from build123d import *

# Parameters (mm, degrees)
F1_DEPTH = 12.7
F2_R     = 5.08
F4_D     = 25.4
F4_DEPTH = 6.35
F4_TIP   = 7.6309298617


# Not quite as in the source:
# - a feature names something its author has since deleted; it is built from what else it names


with BuildPart() as f1:
    # F0 (on Right) → F1 (new body)
    with BuildSketch(Plane.YZ):
        with BuildLine():
            ThreePointArc((-15.875, 0), (0, -15.875), (15.875, 0))
            ThreePointArc((15.875, 0), (0, 15.875), (-15.875, 0))
        make_face()
        with BuildLine():
            Line((15.875, -50.8), (15.875, 0))
            ThreePointArc((15.875, 0), (0, -15.875), (-15.875, 0))
            Line((-15.875, 0), (-15.875, -50.8))
            ThreePointArc((-15.875, -50.8), (0, -34.925), (15.875, -50.8))
        make_face()
        with BuildLine():
            ThreePointArc((-15.875, -50.8), (0, -66.675), (15.875, -50.8))
            ThreePointArc((15.875, -50.8), (0, -34.925), (-15.875, -50.8))
        make_face()
    extrude(amount=F1_DEPTH)

    # F2
    f2_edges = [f1.edges().sort_by_distance(p)[0] for p in [
        (12.7, 0, 15.875),
        (12.7, -15.875, -25.4),
        (12.7, 0, -66.675),
        (12.7, 15.875, -25.4),
    ]]
    fillet(f2_edges, radius=F2_R)

    # F4
    with Locations(Plane(origin=(0, 0, 0), x_dir=(0, -1, 0), z_dir=(-1, 0, 0))):
        with Locations((0, 0)):
            Hole(F4_D / 2, depth=F4_DEPTH)
            with Locations((0, 0, -(F4_DEPTH + F4_TIP / 2))):  # 118° drill point
                Cone(0, F4_D / 2, F4_TIP, mode=Mode.SUBTRACT)


solid = f1.part
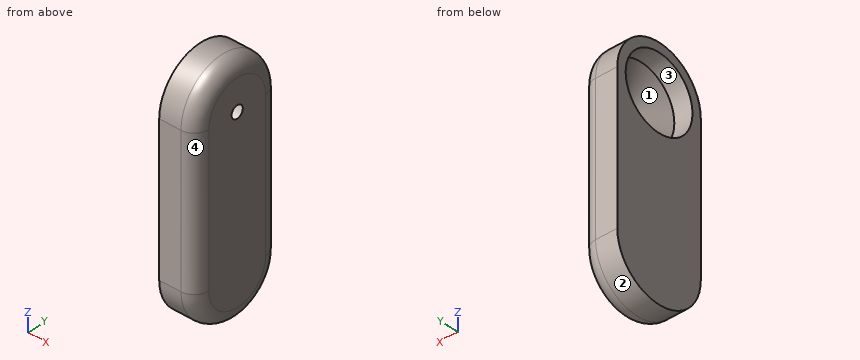
The listing builds one solid part. Answer for the finished solid, in the listing's coordinates (mm). Face numbers are marked on the shaded views. Round coordinates to 2 decimals unless told otherwise and drop trailing zeros. Order: outer loops, then holes, each group sorted by start corner. A loop starts at its lowest first (then second) coordinate and runs counter-clockwise, first axis right, second up. Notation, with made-up numbers: (34.25, 64.5) - (68.25, 64.5) arc R19 cw to (68.25, 100.5) - close; hole circle Ø11 at (88, 46.25). An arc over 180 degrees is marked (long way). Write item = value, one per line. Start each with the question number.
1) Given pin 1 (3 mm diameter, centred on x = 9, y = -3, fed in from -Z); pin 2 (5 mm diameter, centred on x = 8.5, y = 0, fed in from +Z) (3 decimals); pin 3 (4 mm diameter, centred on x = 10.5, z = -33, fed in from +Y), each flat-ended and moving along its own axis, determine where each tip first touches the part or whether it passes through.
2) Section B-B, the plane z = -40 is taken. Write down the section's boundary in (x, y) (3 decimals).
3) Straight lines are drawn through the part: L1, parallel to Y at x = 3, z = 0 (3 decimals); L2, parallel to Z at x = 4.5, y = 0 (3 decimals); L3, parallel to Y at x = 8, z = 2.5. For each, find the intervals that lie inside material, in ascending order.
4) Section D-D, the plane x = 10 is taken. Write down the section's boundary in (y, z).
5) Section A-A, the plane x = 4.5 is taken. Write down the section's boundary in (y, z) (3 decimals), plus the area to 3 significant figures.
6) Section C-C, the plane y = 0 is taken. Write down the section's boundary in (x, z) (3 decimals), plus the area to 3 significant figures.
7) For a pull along Z with two mould halves and no side action, classify the marked faces 1, 2, 3 and 4 as released by +Z, released by -Z, zero draft, split by the parting line, or undercut.
Results list:
q1.pin_1 = -66.55
q1.pin_2 = 15.875
q1.pin_3 = 15.8
q2.outline = (0, -15.875) - (7.62, -15.875) arc R5.08 ccw to (12.7, -10.795) - (12.7, 10.795) arc R5.08 ccw to (7.62, 15.875) - (0, 15.875) - close
q3.L1 = -15.875 to -12.7, 12.7 to 15.875
q3.L2 = -66.675 to -12.7, 12.7 to 15.875
q3.L3 = -15.66 to -9.63, 9.63 to 15.66
q4.outline = (-15.28, -50.8) arc R15.28 ccw to (15.28, -50.8) - (15.28, 0) arc R15.28 ccw to (-15.28, 0) - close; hole circle Ø13.25 at (0, 0)
q5.outline = (-15.875, -50.8) arc R15.875 ccw to (15.875, -50.8) - (15.875, 0) arc R15.875 ccw to (-15.875, 0) - close; hole circle Ø25.4 at (0, 0)
q5.area = 1,900 mm^2
q6.outline = (0, -66.675) - (7.62, -66.675) arc R5.08 ccw to (12.7, -61.595) - (12.7, -2.132) - (6.35, -12.7) - (0, -12.7) - close; (0, 12.7) - (6.35, 12.7) - (12.7, 2.132) - (12.7, 10.795) arc R5.08 ccw to (7.62, 15.875) - (0, 15.875) - close
q6.area = 782 mm^2
q7.face_1 = undercut
q7.face_2 = released by -Z
q7.face_3 = undercut
q7.face_4 = zero draft
